Could you check a few things on this model? Use its own coordinates, in mm. Round coordinates to 2 decimals unless told otherwise and drop trailing zeros. Write each loop counter-clockwise with the first axis right and the second up, starting at its lowest first coordinate (ties: lowest second). Pieces come first, ordered by that corner, then holes. Notation, with made-up numbers: M 86,-18 L 131,-18 A14 ccw 131,4 Z; hole C 56,-36.75 d6. An arc over 180 degrees is marked long. One line per item, written item: value. Start each with the question number.
(1) I want a section at C-C on x = -27.5. Please give me the cut outline in (y, z).
(2) I'm going to push flat-ended pins straight in: pin 1 Ø1 at (y, z) = (37.5, -21.5) entering from -X; pin 2 Ø1.5 at (x, y) = (-103.5, 38) entering from -Z; pin 3 Ø10 at (x, z) = (-34.5, 65) entering from -Y; pin 4 Ø1 at (y, z) = (37, 48.5) entering from +X. Where does each tip first touch, or does it pass through?
(3) Thinking about a two-plate mould opening in Z: for faces 1 (the face through (-77, 35.867, -1)), 2 (the face through (-88.1, 37.5, -1.9)), 3 (the face through (-35.346, 37.433, -57.79)), which applies, released by +Z, released by -Z, zero draft, split by the parting line, or undercut?
(4) I want a section at A-A on z = -69. Please give me the cut outline in (x, y), and give its area (3 significant figures).
(5) I want a section at B-B on y = 37.45. Please give me the cut outline in (x, z).
(6) I want a section at D-D on z = 17.5. Please give me the cut outline in (x, y), and give its area (3 significant figures).
(7) If I drill on L1, parallel to X at y = 38.15, z = 0; L2, parallel to Z at x = -155, y = 38.1; L3, parallel to X at y = 36.1, z = -38.5, over which ranges is the centre line in solid material (lowest first)?
```python
from build123d import *

# Parameters (mm, degrees)
BOSS_EXTRUDE1_DEPTH = 3.175
CUT_EXTRUDE1_REACH  = 5.175
SKETCH5_R           = 6.477


with BuildPart() as part:
    # Sketch4 → Boss-Extrude1 (new body)
    with BuildSketch(Plane(origin=(0, 35.86734, 0), x_dir=(1, 0, 0), z_dir=(0, 1, 0))):
        with BuildLine():
            Line((-176.599307952, 6.35), (-124.425974424, 6.35))
            ThreePointArc((-124.425974424, 6.35), (-118.075974424, 0), (-124.425974424, -6.35))
            Line((-124.425974424, -6.35), (-176.599307952, -6.35))
            ThreePointArc((-176.599307952, -6.35), (-152.665565869, -58.371664787), (-100.643901082, -82.30540687))
            Line((-100.643901082, -82.30540687), (-100.643901082, -30.132073341))
            ThreePointArc((-100.643901082, -30.132073341), (-94.293901082, -23.782073341), (-87.943901082, -30.132073341))
            Line((-87.943901082, -30.132073341), (-87.943901082, -82.30540687))
            ThreePointArc((-87.943901082, -82.30540687), (-35.922236295, -58.371664787), (-11.988494212, -6.35))
            Line((-11.988494212, -6.35), (-64.161827741, -6.35))
            ThreePointArc((-64.161827741, -6.35), (-70.511827741, 0), (-64.161827741, 6.35))
            Line((-64.161827741, 6.35), (-11.988494212, 6.35))
            ThreePointArc((-11.988494212, 6.35), (-35.922236295, 58.371664787), (-87.943901082, 82.30540687))
            Line((-87.943901082, 82.30540687), (-87.943901082, 30.132073341))
            ThreePointArc((-87.943901082, 30.132073341), (-94.293901082, 23.782073341), (-100.643901082, 30.132073341))
            Line((-100.643901082, 30.132073341), (-100.643901082, 82.30540687))
            ThreePointArc((-100.643901082, 82.30540687), (-152.665565869, 58.371664787), (-176.599307952, 6.35))
        make_face()
    extrude(amount=BOSS_EXTRUDE1_DEPTH)

    # Sketch5 → Cut-Extrude1 (cut, up to next)
    with BuildSketch(Plane(origin=(0, 39.04234, 0), x_dir=(1, 0, 0), z_dir=(0, 1, 0)), mode=Mode.PRIVATE) as cut_extrude1_sk1:
        with Locations((-94.293901082, 0)):
            Circle(SKETCH5_R)
    cut_extrude1_tool1 = extrude(cut_extrude1_sk1.sketch, amount=-CUT_EXTRUDE1_REACH, mode=Mode.PRIVATE) & part.part
    add(cut_extrude1_tool1.solids().sort_by_distance((-94.293901, 39.04234, 0))[0], mode=Mode.SUBTRACT)


solid = part.part
```
Found:
1. outline: M 35.87,-48.51 L 39.04,-48.51 L 39.04,-6.35 L 35.87,-6.35 Z; M 35.87,6.35 L 39.04,6.35 L 39.04,48.51 L 35.87,48.51 Z
2. pin 1: stops at x = -174.13
2. pin 2: stops at z = -82.12
2. pin 3: passes through
2. pin 4: stops at x = -27.13
3. face 1: zero draft
3. face 2: undercut
3. face 3: released by -Z
4. outline: M -139.61,35.87 L -100.64,35.87 L -100.64,39.04 L -139.61,39.04 Z; M -87.94,35.87 L -48.98,35.87 L -48.98,39.04 L -87.94,39.04 Z
4. area: 247 mm²
5. outline: M -176.6,-6.35 A82.55 ccw -100.64,-82.31 L -100.64,-30.13 A6.35 cw -87.94,-30.13 L -87.94,-82.31 A82.55 ccw -11.99,-6.35 L -64.16,-6.35 A6.35 cw -64.16,6.35 L -11.99,6.35 A82.55 ccw -87.94,82.31 L -87.94,30.13 A6.35 cw -100.64,30.13 L -100.64,82.31 A82.55 ccw -176.6,6.35 L -124.43,6.35 A6.35 cw -124.43,-6.35 Z; hole C -94.29,0 d12.95
6. outline: M -174.97,35.87 L -13.62,35.87 L -13.62,39.04 L -174.97,39.04 Z
6. area: 512 mm²
7. L1: x = -118.08 to -100.77, -87.82 to -70.51
7. L2: z = -55.94 to -6.35, 6.35 to 55.94
7. L3: x = -167.32 to -100.64, -87.94 to -21.27
